Geometry check sheet. Reference: the model listing, model coordinates, mm. A direction names the side the tool comes from. Round coordinates to 2 decimals unless told otherwise and drop trailing zeros. Order: outer loops, then holes, each group sorted by start corner. A loop starts at its lowest first (then second) coordinate and runs counter-clockwise, first axis right, second up.
```python
from build123d import *

# Parameters (mm, degrees)
SKETCH_1_W           = 200
SKETCH_1_H           = 150
EXTRUDE_1_DEPTH      = 5
SKETCH_2_W           = 280
SKETCH_2_H           = 250
SKETCH_2_R           = 1.5
EXTRUDE_2_DEPTH      = 5
SKETCH_3_R           = 11.5
CUT_EXTRUDE_1_DEPTH  = 5
SKETCH_4_R           = 3
SKETCH_4_R_2         = 1.5
EXTRUDE_3_DEPTH      = 13
CUT_EXTRUDE_4_REACH  = 190.133
SKETCH_8_R           = 1.5
CUT_EXTRUDE_5_REACH  = 190.133
SKETCH_9_W           = 10
SKETCH_9_H           = 250
SKETCH_10_W          = 41.454704644
SKETCH_10_H          = 62.998147515
CUT_EXTRUDE_6_DEPTH  = 13
CUT_EXTRUDE_7_REACH  = 182.416
SKETCH_11_R          = 1.5
CUT_EXTRUDE_8_DEPTH  = 2
CUT_EXTRUDE_9_REACH  = 182.416
SKETCH_13_R          = 30
CUT_EXTRUDE_10_REACH = 182.416
SKETCH_17_R          = 4
CUT_EXTRUDE_11_DEPTH = 2.5
SKETCH_18_W          = 49
SKETCH_18_H          = 49
SKETCH_18_W_2        = 45
SKETCH_18_H_2        = 45
CUT_EXTRUDE_12_DEPTH = 2
SKETCH_19_R          = 1.5
CUT_EXTRUDE_13_DEPTH = 2


# Read off the part's stored shape, not the designer's step: 旋转4
with BuildPart() as part:
    # 草图1 → 凸台-拉伸1 (new body)
    with BuildSketch(Plane(origin=(0, 0, 0), x_dir=(1, 0, 0), z_dir=(0, 1, 0))):
        Rectangle(SKETCH_1_W, SKETCH_1_H)
    extrude(amount=EXTRUDE_1_DEPTH)

    # 草图2 → 凸台-拉伸2 (add)
    with BuildSketch(Plane(origin=(0, 5, 0), x_dir=(1, 0, 0), z_dir=(0, 1, 0))):
        Rectangle(SKETCH_2_W, SKETCH_2_H)
        with Locations(Location((-105, 70, 0), (0, 0, 270))):
            Circle(SKETCH_2_R, mode=Mode.SUBTRACT)
        with Locations(Location((-105, -70, 0), (0, 0, 270))):
            Circle(SKETCH_2_R, mode=Mode.SUBTRACT)
        with Locations(Location((105, 70, 0), (0, 0, 270))):
            Circle(SKETCH_2_R, mode=Mode.SUBTRACT)
        with Locations(Location((105, -70, 0), (0, 0, 270))):
            Circle(SKETCH_2_R, mode=Mode.SUBTRACT)
    extrude(amount=-EXTRUDE_2_DEPTH)

    # 草图3 → 切除-拉伸1 (cut)
    with BuildSketch(Plane(origin=(0, 5, 0), x_dir=(1, 0, 0), z_dir=(0, 1, 0))):
        with Locations(Location((0, -85, 0), (0, 0, 270))):
            Circle(SKETCH_3_R)
    extrude(amount=-CUT_EXTRUDE_1_DEPTH, mode=Mode.SUBTRACT)

    # 草图4 → 凸台-拉伸3 (add)
    # profile 1 of 4: a face of its own
    with BuildSketch(Plane.XZ):
        with Locations(Location((-5, 119.8, 0), (0, 0, 90))):
            Circle(SKETCH_4_R)
        with Locations(Location((-5, 119.8, 0), (0, 0, 90))):
            Circle(SKETCH_4_R_2, mode=Mode.SUBTRACT)
    # profile 2 of 4: a face of its own
    with BuildSketch(Plane.XZ):
        with Locations(Location((5, 119.8, 0), (0, 0, 90))):
            Circle(SKETCH_4_R)
        with Locations(Location((5, 119.8, 0), (0, 0, 90))):
            Circle(SKETCH_4_R_2, mode=Mode.SUBTRACT)
    # profile 3 of 4: a face of its own
    with BuildSketch(Plane.XZ):
        with Locations(Location((5, 70.2, 0), (0, 0, 90))):
            Circle(SKETCH_4_R)
        with Locations(Location((5, 70.2, 0), (0, 0, 90))):
            Circle(SKETCH_4_R_2, mode=Mode.SUBTRACT)
    # profile 4 of 4: a face of its own
    with BuildSketch(Plane.XZ):
        with Locations(Location((-5, 70.2, 0), (0, 0, 90))):
            Circle(SKETCH_4_R)
        with Locations(Location((-5, 70.2, 0), (0, 0, 90))):
            Circle(SKETCH_4_R_2, mode=Mode.SUBTRACT)
    extrude(amount=EXTRUDE_3_DEPTH)

    # 草图8 → 切除-拉伸4 (cut, up to next)
    with BuildSketch(Plane.XZ, mode=Mode.PRIVATE) as cut_extrude_4_sk1:
        with Locations(Location((5, 119.8, 0), (0, 0, 90))):
            Circle(SKETCH_8_R)
    cut_extrude_4_tool1 = extrude(cut_extrude_4_sk1.sketch, amount=-CUT_EXTRUDE_4_REACH, mode=Mode.PRIVATE) & part.part
    # 草图8 → 切除-拉伸4 (cut, up to next)
    with BuildSketch(Plane.XZ, mode=Mode.PRIVATE) as cut_extrude_4_sk2:
        with Locations(Location((5, 70.2, 0), (0, 0, 90))):
            Circle(SKETCH_8_R)
    cut_extrude_4_tool2 = extrude(cut_extrude_4_sk2.sketch, amount=-CUT_EXTRUDE_4_REACH, mode=Mode.PRIVATE) & part.part
    # 草图8 → 切除-拉伸4 (cut, up to next)
    with BuildSketch(Plane.XZ, mode=Mode.PRIVATE) as cut_extrude_4_sk3:
        with Locations(Location((-5, 119.8, 0), (0, 0, 90))):
            Circle(SKETCH_8_R)
    cut_extrude_4_tool3 = extrude(cut_extrude_4_sk3.sketch, amount=-CUT_EXTRUDE_4_REACH, mode=Mode.PRIVATE) & part.part
    # 草图8 → 切除-拉伸4 (cut, up to next)
    with BuildSketch(Plane.XZ, mode=Mode.PRIVATE) as cut_extrude_4_sk4:
        with Locations(Location((-5, 70.2, 0), (0, 0, 90))):
            Circle(SKETCH_8_R)
    cut_extrude_4_tool4 = extrude(cut_extrude_4_sk4.sketch, amount=-CUT_EXTRUDE_4_REACH, mode=Mode.PRIVATE) & part.part
    add(cut_extrude_4_tool1.solids().sort_by_distance((5, 0, 119.8))[0], mode=Mode.SUBTRACT)
    add(cut_extrude_4_tool2.solids().sort_by_distance((5, 0, 70.2))[0], mode=Mode.SUBTRACT)
    add(cut_extrude_4_tool3.solids().sort_by_distance((-5, 0, 119.8))[0], mode=Mode.SUBTRACT)
    add(cut_extrude_4_tool4.solids().sort_by_distance((-5, 0, 70.2))[0], mode=Mode.SUBTRACT)

    # 草图9 → 切除-拉伸5 (cut, up to next)
    with BuildSketch(Plane.XZ, mode=Mode.PRIVATE) as cut_extrude_5_sk1:
        with Locations((-135, 0)):
            Rectangle(SKETCH_9_W, SKETCH_9_H)
    cut_extrude_5_tool1 = extrude(cut_extrude_5_sk1.sketch, amount=-CUT_EXTRUDE_5_REACH, mode=Mode.PRIVATE) & part.part
    # 草图9 → 切除-拉伸5 (cut, up to next)
    with BuildSketch(Plane.XZ, mode=Mode.PRIVATE) as cut_extrude_5_sk2:
        with Locations((135, 0)):
            Rectangle(SKETCH_9_W, SKETCH_9_H)
    cut_extrude_5_tool2 = extrude(cut_extrude_5_sk2.sketch, amount=-CUT_EXTRUDE_5_REACH, mode=Mode.PRIVATE) & part.part
    add(cut_extrude_5_tool1.solids().sort_by_distance((-135, 0, 0))[0], mode=Mode.SUBTRACT)
    add(cut_extrude_5_tool2.solids().sort_by_distance((135, 0, 0))[0], mode=Mode.SUBTRACT)

    # 草图10 → 切除-拉伸6 (cut)
    with BuildSketch(Plane.XZ):
        with Locations((1.571094054, 93.500926243)):
            Rectangle(SKETCH_10_W, SKETCH_10_H)
    extrude(amount=CUT_EXTRUDE_6_DEPTH, mode=Mode.SUBTRACT)

    # 草图11 → 切除-拉伸7 (cut, up to next)
    with BuildSketch(Plane(origin=(0, 5, 0), x_dir=(1, 0, 0), z_dir=(0, 1, 0)), mode=Mode.PRIVATE) as cut_extrude_7_sk1:
        with Locations(Location((-18.68, 121.18, 0), (0, 0, 270))):
            Circle(SKETCH_11_R)
    cut_extrude_7_tool1 = extrude(cut_extrude_7_sk1.sketch, amount=-CUT_EXTRUDE_7_REACH, mode=Mode.PRIVATE) & part.part
    # 草图11 → 切除-拉伸7 (cut, up to next)
    with BuildSketch(Plane(origin=(0, 5, 0), x_dir=(1, 0, 0), z_dir=(0, 1, 0)), mode=Mode.PRIVATE) as cut_extrude_7_sk2:
        with Locations(Location((18.68, 121.18, 0), (0, 0, 270))):
            Circle(SKETCH_11_R)
    cut_extrude_7_tool2 = extrude(cut_extrude_7_sk2.sketch, amount=-CUT_EXTRUDE_7_REACH, mode=Mode.PRIVATE) & part.part
    # 草图11 → 切除-拉伸7 (cut, up to next)
    with BuildSketch(Plane(origin=(0, 5, 0), x_dir=(1, 0, 0), z_dir=(0, 1, 0)), mode=Mode.PRIVATE) as cut_extrude_7_sk3:
        with Locations(Location((18.68, 83.82, 0), (0, 0, 270))):
            Circle(SKETCH_11_R)
    cut_extrude_7_tool3 = extrude(cut_extrude_7_sk3.sketch, amount=-CUT_EXTRUDE_7_REACH, mode=Mode.PRIVATE) & part.part
    # 草图11 → 切除-拉伸7 (cut, up to next)
    with BuildSketch(Plane(origin=(0, 5, 0), x_dir=(1, 0, 0), z_dir=(0, 1, 0)), mode=Mode.PRIVATE) as cut_extrude_7_sk4:
        with Locations(Location((-18.68, 83.82, 0), (0, 0, 270))):
            Circle(SKETCH_11_R)
    cut_extrude_7_tool4 = extrude(cut_extrude_7_sk4.sketch, amount=-CUT_EXTRUDE_7_REACH, mode=Mode.PRIVATE) & part.part
    add(cut_extrude_7_tool1.solids().sort_by_distance((-18.68, 5, -121.18))[0], mode=Mode.SUBTRACT)
    add(cut_extrude_7_tool2.solids().sort_by_distance((18.68, 5, -121.18))[0], mode=Mode.SUBTRACT)
    add(cut_extrude_7_tool3.solids().sort_by_distance((18.68, 5, -83.82))[0], mode=Mode.SUBTRACT)
    add(cut_extrude_7_tool4.solids().sort_by_distance((-18.68, 5, -83.82))[0], mode=Mode.SUBTRACT)

    # 草图12 → 切除-拉伸8 (cut)
    with BuildSketch(Plane(origin=(0, 5, 0), x_dir=(1, 0, 0), z_dir=(0, 1, 0))):
        Polygon((-23.5, 79), (23.5, 79), (23.5, 125), (25.5, 125), (25.5, 77), (-25.5, 77), (-25.5, 125), (-23.5, 125), align=None)
    extrude(amount=-CUT_EXTRUDE_8_DEPTH, mode=Mode.SUBTRACT)

    # 草图13 → 切除-拉伸9 (cut, up to next)
    with BuildSketch(Plane(origin=(0, 5, 0), x_dir=(1, 0, 0), z_dir=(0, 1, 0)), mode=Mode.PRIVATE) as cut_extrude_9_sk1:
        with Locations(Location((0, 0, 0), (0, 0, 270))):
            Circle(SKETCH_13_R)
    cut_extrude_9_tool1 = extrude(cut_extrude_9_sk1.sketch, amount=-CUT_EXTRUDE_9_REACH, mode=Mode.PRIVATE) & part.part
    add(cut_extrude_9_tool1.solids().sort_by_distance((0, 5, 0))[0], mode=Mode.SUBTRACT)

    # 草图14 → 切除-拉伸10 (cut, up to next)
    with BuildSketch(Plane(origin=(0, 5, 0), x_dir=(1, 0, 0), z_dir=(0, 1, 0)), mode=Mode.PRIVATE) as cut_extrude_10_sk1:
        with BuildLine():
            Line((77.75, 125), (130, 125))
            Line((130, 125), (130, 69.065639069))
            ThreePointArc((130, 69.065639069), (107.574061968, 100.488226633), (77.75, 125))
        make_face()
    cut_extrude_10_tool1 = extrude(cut_extrude_10_sk1.sketch, amount=-CUT_EXTRUDE_10_REACH, mode=Mode.PRIVATE) & part.part
    # 草图14 → 切除-拉伸10 (cut, up to next)
    with BuildSketch(Plane(origin=(0, 5, 0), x_dir=(1, 0, 0), z_dir=(0, 1, 0)), mode=Mode.PRIVATE) as cut_extrude_10_sk2:
        with BuildLine():
            Line((77.75, -125), (130, -125))
            Line((130, -125), (130, -69.065639069))
            ThreePointArc((130, -69.065639069), (107.574061968, -100.488226633), (77.75, -125))
        make_face()
    cut_extrude_10_tool2 = extrude(cut_extrude_10_sk2.sketch, amount=-CUT_EXTRUDE_10_REACH, mode=Mode.PRIVATE) & part.part
    # 草图14 → 切除-拉伸10 (cut, up to next)
    with BuildSketch(Plane(origin=(0, 5, 0), x_dir=(1, 0, 0), z_dir=(0, 1, 0)), mode=Mode.PRIVATE) as cut_extrude_10_sk3:
        with BuildLine():
            Line((-130, -125), (-130, -69.065639069))
            ThreePointArc((-130, -69.065639069), (-107.574061968, -100.488226633), (-77.75, -125))
            Line((-77.75, -125), (-130, -125))
        make_face()
    cut_extrude_10_tool3 = extrude(cut_extrude_10_sk3.sketch, amount=-CUT_EXTRUDE_10_REACH, mode=Mode.PRIVATE) & part.part
    # 草图14 → 切除-拉伸10 (cut, up to next)
    with BuildSketch(Plane(origin=(0, 5, 0), x_dir=(1, 0, 0), z_dir=(0, 1, 0)), mode=Mode.PRIVATE) as cut_extrude_10_sk4:
        with BuildLine():
            Line((-130, 125), (-130, 69.065639069))
            ThreePointArc((-130, 69.065639069), (-107.574061968, 100.488226633), (-77.75, 125))
            Line((-77.75, 125), (-130, 125))
        make_face()
    cut_extrude_10_tool4 = extrude(cut_extrude_10_sk4.sketch, amount=-CUT_EXTRUDE_10_REACH, mode=Mode.PRIVATE) & part.part
    add(cut_extrude_10_tool1.solids().sort_by_distance((114.14156, 5, -108.066894))[0], mode=Mode.SUBTRACT)
    add(cut_extrude_10_tool2.solids().sort_by_distance((114.14156, 5, 108.066894))[0], mode=Mode.SUBTRACT)
    add(cut_extrude_10_tool3.solids().sort_by_distance((-114.14156, 5, 108.066894))[0], mode=Mode.SUBTRACT)
    add(cut_extrude_10_tool4.solids().sort_by_distance((-114.14156, 5, -108.066894))[0], mode=Mode.SUBTRACT)

    # 旋转4 outline → 旋转4 (revolve)
    with BuildSketch(Plane(origin=(-103.875, 0, 0), x_dir=(1, 0, 0), z_dir=(0, 0, 1))):
        with BuildLine():
            Line((0, 4.999999981), (19, 4.999999981))
            ThreePointArc((19, 4.999999981), (13.435028849, 18.435028836), (0, 24))
            Line((0, 24), (0, 4.999999981))
        make_face()
    revolve(axis=Axis((-103.875, 0, 0), (0, 1, 0)))

    # 草图17 → 切除-拉伸11 (cut)
    with BuildSketch(Plane(origin=(0, 5, 0), x_dir=(1, 0, 0), z_dir=(0, 1, 0))):
        with Locations(Location((-105, 70, 0), (0, 0, 270))):
            Circle(SKETCH_17_R)
        with Locations(Location((105, 70, 0), (0, 0, 270))):
            Circle(SKETCH_17_R)
        with Locations(Location((105, -70, 0), (0, 0, 270))):
            Circle(SKETCH_17_R)
        with Locations(Location((-105, -70, 0), (0, 0, 270))):
            Circle(SKETCH_17_R)
    extrude(amount=-CUT_EXTRUDE_11_DEPTH, mode=Mode.SUBTRACT)

    # 草图18 → 切除-拉伸12 (cut)
    with BuildSketch(Plane(origin=(0, 5, 0), x_dir=(1, 0, 0), z_dir=(0, 1, 0))):
        with Locations((100, 0)):
            Rectangle(SKETCH_18_W, SKETCH_18_H)
        with Locations((100, 0)):
            Rectangle(SKETCH_18_W_2, SKETCH_18_H_2, mode=Mode.SUBTRACT)
    extrude(amount=-CUT_EXTRUDE_12_DEPTH, mode=Mode.SUBTRACT)

    # 草图19 → 切除-拉伸13 (cut)
    with BuildSketch(Plane(origin=(0, 5, 0), x_dir=(1, 0, 0), z_dir=(0, 1, 0))):
        with Locations(Location((117.5, 17.5, 0), (0, 0, 270))):
            Circle(SKETCH_19_R)
        with Locations(Location((82.5, 17.5, 0), (0, 0, 270))):
            Circle(SKETCH_19_R)
        with Locations(Location((117.5, -17.5, 0), (0, 0, 270))):
            Circle(SKETCH_19_R)
        with Locations(Location((82.5, -17.5, 0), (0, 0, 270))):
            Circle(SKETCH_19_R)
        with Locations(Location((100, 0, 0), (0, 0, 270))):
            Circle(SKETCH_19_R)
    extrude(amount=-CUT_EXTRUDE_13_DEPTH, mode=Mode.SUBTRACT)


solid = part.part
```
(1) Sectioned sample at C-C, the plane y = 9. Record the cut outline in (x, z) (3 decimals), and give its area (3 significant figures).
Returned:
outline: circle Ø37.148 at (-103.875, 0)
area: 1,080 mm2
(2) Draft check along Z on faces 4 (the cylindrical face through (107.943, 2.535, 100.091)), 5 (the flat face through (0, 5, -102)), 6 (the cylindrical face through (-106.532, 3.768, 73.695)), 7 (the cylindrical face through (103.468, 3.768, 73.695)). Enter one of: released by +Z, released by -Z, zero draft, split by the parting line, or undercut.
Returned:
face 4: released by +Z
face 5: zero draft
face 6: undercut
face 7: undercut
(3) Sectioned sample at B-B, the plane z = -36. Record the cut outline in (x, y).
Returned:
outline: (-130, 0) - (130, 0) - (130, 5) - (-130, 5) - close
(4) Sectioned sample at A-A, the plane x = -47. Record the cut outline in (y, z).
Returned:
outline: (0, -125) - (5, -125) - (5, 125) - (0, 125) - close
(5) Depth check by flat-ended pin: P1, Ø1.6, axis at y = 4.5, z = -106.5, coming from the +X side; P2, Ø10, axis at x = -94.5, z = 4, coming from the +Y side; P3, Ø3.5, axis at x = 82, z = 18, coming from the +Y side; P4, Ø10, axis at y = 12.5, z = -99, coming from the -X side. Enter the tip coordinate at first touch or a pass-through.
Returned:
P1: stops at x = 102.46
P2: stops at y = 23.28
P3: stops at y = 5
P4: passes through
(6) Material ranges on line 1 (X direction, y = 3.45, z = 0); line 2 (X direction, y = 2.85, z = 119.8); line 3 (X direction, y = 3.85, z = -70), recorded low to high.
Returned:
line 1: x = -130 to -30, 30 to 75.5, 77.5 to 98.5, 101.5 to 122.5, 124.5 to 130
line 2: x = -85.55 to -6.5, -3.5 to 3.5, 6.5 to 85.55
line 3: x = -129.5 to -109, -101 to 101, 109 to 129.5
(7) Set-up check for faces 1 (the cylindrical face through (-107.943, 2.535, -100.091)), 2 (the flat face through (103, 2.5, 70)), 3 (the flat face through (105, 5, 0)): record each of +Z, -Z, +X, -X, +Y, -Y from which the full face is reachable in a straight line by a thin tool's end or side.
Returned:
face 1: -Z, -X, +Y, -Y
face 2: +Y
face 3: +Z, -Z, +X, +Y
